from build123d import *

# Parameters (mm, degrees)
CROQUIS1_R                   = 7.65
SALIENTE_EXTRUIR1_DEPTH      = 8.5
CROQUIS2_R                   = 7.65
CROQUIS2_R_2                 = 5
SALIENTE_EXTRUIR2_DEPTH      = 21.5
SALIENTE_EXTRUIR3_REACH      = 132.896
SALIENTE_EXTRUIR3_END_RADIUS = 7.65
SALIENTE_EXTRUIR3_START      = 12
CROQUIS3_R                   = 6.5
CORTAR_EXTRUIR1_REACH        = 129.309
CORTAR_EXTRUIR1_END_RADIUS   = 5
CROQUIS4_R                   = 2.25


with BuildPart() as part:
    # Croquis1 → Saliente-Extruir1 (new, symmetric)
    with BuildSketch(Plane(origin=(0, 0, 0), x_dir=(1, 0, 0), z_dir=(0, 1, 0))):
        with BuildLine():
            ThreePointArc((-18.62950636, 70.733830846), (-21.266037972, 78.379045573), (-29.224003483, 79.818278736))
            ThreePointArc((-29.224003483, 79.818278736), (-42.5, 73.612159322), (-54.51265533, 65.217868785))
            ThreePointArc((-54.51265533, 65.217868785), (-57.245225604, 57.606451909), (-51.942541239, 51.500541191))
            ThreePointArc((-51.942541239, 51.500541191), (-41.569219382, 24), (-70.572047599, 19.233289655))
            ThreePointArc((-70.572047599, 19.233289655), (-78.511263577, 20.772593665), (-83.736658814, 14.600409951))
            ThreePointArc((-83.736658814, 14.600409951), (-85, 0), (-83.736658814, -14.600409951))
            ThreePointArc((-83.736658814, -14.600409951), (-78.511263577, -20.772593665), (-70.572047599, -19.233289655))
            ThreePointArc((-70.572047599, -19.233289655), (-41.569219382, -24), (-51.942541239, -51.500541191))
            ThreePointArc((-51.942541239, -51.500541191), (-57.245225604, -57.606451909), (-54.51265533, -65.217868785))
            ThreePointArc((-54.51265533, -65.217868785), (-42.5, -73.612159322), (-29.224003483, -79.818278736))
            ThreePointArc((-29.224003483, -79.818278736), (-21.266037972, -78.379045573), (-18.62950636, -70.733830846))
            ThreePointArc((-18.62950636, -70.733830846), (0, -48), (18.62950636, -70.733830846))
            ThreePointArc((18.62950636, -70.733830846), (21.266037972, -78.379045573), (29.224003483, -79.818278736))
            ThreePointArc((29.224003483, -79.818278736), (42.5, -73.612159322), (54.51265533, -65.217868785))
            ThreePointArc((54.51265533, -65.217868785), (57.245225604, -57.606451909), (51.942541239, -51.500541191))
            ThreePointArc((51.942541239, -51.500541191), (41.569219382, -24), (70.572047599, -19.233289655))
            ThreePointArc((70.572047599, -19.233289655), (78.511263577, -20.772593665), (83.736658814, -14.600409951))
            ThreePointArc((83.736658814, -14.600409951), (85, 0), (83.736658814, 14.600409951))
            ThreePointArc((83.736658814, 14.600409951), (78.511263577, 20.772593665), (70.572047599, 19.233289655))
            ThreePointArc((70.572047599, 19.233289655), (41.569219382, 24), (51.942541239, 51.500541191))
            ThreePointArc((51.942541239, 51.500541191), (57.245225604, 57.606451909), (54.51265533, 65.217868785))
            ThreePointArc((54.51265533, 65.217868785), (42.5, 73.612159322), (29.224003483, 79.818278736))
            ThreePointArc((29.224003483, 79.818278736), (21.266037972, 78.379045573), (18.62950636, 70.733830846))
            ThreePointArc((18.62950636, 70.733830846), (0, 48), (-18.62950636, 70.733830846))
        make_face()
        with Locations(Location((0, 0, 0), (0, 0, 270))):
            Circle(CROQUIS1_R, mode=Mode.SUBTRACT)
    extrude(amount=SALIENTE_EXTRUIR1_DEPTH, both=True)


with BuildPart() as body_2:
    # Croquis2 → Saliente-Extruir2 (new body)
    with BuildSketch(Plane(origin=(0, 0, 0), x_dir=(1, 0, 0), z_dir=(0, 1, 0))):
        with Locations(Location((0, 0, 0), (0, 0, 270))):
            Circle(CROQUIS2_R)
        with Locations(Location((0, 0, 0), (0, 0, 270))):
            Circle(CROQUIS2_R_2, mode=Mode.SUBTRACT)
    extrude(amount=SALIENTE_EXTRUIR2_DEPTH)

    # Simetría3: body 2 across plane


with BuildPart() as body_2_1:
    add(body_2.part)
    add(body_2.part.mirror(Plane.ZX))

    # Saliente-Extruir3: up to this cylinder (the profile starts outside it)
    saliente_extruir3_end = Plane(origin=(0, 15, 0), z_dir=(0, -1, 0)) * Cylinder(SALIENTE_EXTRUIR3_END_RADIUS, 282.092, mode=Mode.PRIVATE)
    # Croquis3 → Saliente-Extruir3 (add, up to the surface)
    with BuildSketch(Plane.XY.offset(SALIENTE_EXTRUIR3_START), mode=Mode.PRIVATE) as saliente_extruir3_sk1:
        with Locations((0, 15)):
            Circle(CROQUIS3_R)
        Polygon((0, 10.958548116), (3.5, 12.979274058), (3.5, 17.020725942), (0, 19.041451884), (-3.5, 17.020725942), (-3.5, 12.979274058), align=None, mode=Mode.SUBTRACT)
    saliente_extruir3_tool1 = extrude(saliente_extruir3_sk1.sketch, amount=-SALIENTE_EXTRUIR3_REACH, mode=Mode.PRIVATE) - saliente_extruir3_end
    add(saliente_extruir3_tool1.solids().sort_by_distance((-6.316152, 15, 12))[0])

    # Cortar-Extruir1: up to this cylinder (the profile starts outside it)
    cortar_extruir1_end = Plane(origin=(0, 15, 0), z_dir=(0, -1, 0)) * Cylinder(CORTAR_EXTRUIR1_END_RADIUS, 269.618, mode=Mode.PRIVATE)
    # Croquis4 → Cortar-Extruir1 (cut, up to the surface)
    with BuildSketch(Plane.XY.offset(12), mode=Mode.PRIVATE) as cortar_extruir1_sk1:
        with Locations((0, 15)):
            Circle(CROQUIS4_R)
    cortar_extruir1_tool1 = extrude(cortar_extruir1_sk1.sketch, amount=-CORTAR_EXTRUIR1_REACH, mode=Mode.PRIVATE) - cortar_extruir1_end
    add(cortar_extruir1_tool1.solids().sort_by_distance((0, 15, 12))[0], mode=Mode.SUBTRACT)


solid = part.part
Here's how the part is built. I have some questions about the finished solid (model axes, mm). Coordinates: 2 decimals unless noted, no trailing zeros. Order: outer loops, then holes, each group sorted by start corner. A loop starts at its lowest first (then second) coordinate and runs counter-clockwise, first axis right, second up. Notation, with made-up numbers: M -20.75,25.25 L 31.25,25.25 A18 cw 31.25,49.25 Z; hole C 75.5,-13 d11. An arc over 180 degrees is marked long. Answer as CSV lines item,"result".
Item 1: Imagine slicing it at A-A on z = 0. Write out the boundary of the cut face in (x, y).
Results found:
outline,"M -85,-8.5 L -7.65,-8.5 L -7.65,8.5 L -85,8.5 Z; M 7.65,-8.5 L 85,-8.5 L 85,8.5 L 7.65,8.5 Z"
Item 2: We'd pull the mould along X, two halves only. Please class faces 1 (the face through (-42.68, 0.12, 73.51)), 2 (the face through (42.322, 0.119, 73.715)), 3 (the face through (0, 0, -48)): +X half, -X half, draft (parallel to the pull), parting line (faces both ways), or undercut.
Results found:
face 1,"-X half"
face 2,"+X half"
face 3,"undercut"
Item 3: For pin 1 (5 mm diameter, centred on x = 13.5, y = 6, fed in from -Z); pin 2 (23 mm diameter, centred on x = 0, z = 67, fed in from +Y); pin 3 (8 mm diameter, centred on y = 3, z = -18, fed in from -X); pin 4 (1.5 mm diameter, centred on y = -2, z = 45, fed in from +X), each with a flat end and sliding along its axis, tell me the tip position at first contact or that it passes through.
Results found:
pin 1,"z = -56.75"
pin 2,"through"
pin 3,"x = -83.84"
pin 4,"x = 43.5"
Item 4: Imagine slicing it at B-B on x = 0. Write out the boundary of the cut face in (y, z).
Results found:
outline,"M -8.5,-48 L 8.5,-48 L 8.5,-7.65 L -8.5,-7.65 Z; M -8.5,7.65 L 8.5,7.65 L 8.5,48 L -8.5,48 Z"
Item 5: Imagine slicing it at C-C on x = -42. Write out the boundary of the cut face in (y, z), plus the area to 3 significant figures.
Results found:
outline,"M -8.5,-73.9 L 8.5,-73.9 L 8.5,-43.71 L -8.5,-43.71 Z; M -8.5,-23.29 L 8.5,-23.29 L 8.5,23.29 L -8.5,23.29 Z; M -8.5,43.71 L 8.5,43.71 L 8.5,73.9 L -8.5,73.9 Z"
area,"1,820 mm2"
Item 6: Imagine slicing it at D-D on y = 5.75. Write out the boundary of the cut face in (x, z).
Results found:
outline,"M -83.74,-14.6 A8 ccw -70.57,-19.23 A19 cw long -51.94,-51.5 A8 ccw -54.51,-65.22 A85 ccw -29.22,-79.82 A8 ccw -18.63,-70.73 A19 cw long 18.63,-70.73 A8 ccw 29.22,-79.82 A85 ccw 54.51,-65.22 A8 ccw 51.94,-51.5 A19 cw long 70.57,-19.23 A8 ccw 83.74,-14.6 A85 ccw 83.74,14.6 A8 ccw 70.57,19.23 A19 cw long 51.94,51.5 A8 ccw 54.51,65.22 A85 ccw 29.22,79.82 A8 ccw 18.63,70.73 A19 cw long -18.63,70.73 A8 ccw -29.22,79.82 A85 ccw -54.51,65.22 A8 ccw -51.94,51.5 A19 cw long -70.57,19.23 A8 ccw -83.74,14.6 A85 ccw Z; hole C 0,0 d15.3"
Item 7: If I drill on line 1 (Z direction, x = 0.5, y = 1); line 2 (Z direction, x = 50.5, y = 7.5); line 3 (Z direction, x = 43.5, y = 0.5), over which ranges is the centre line in solid material (lowest first)?
Results found:
line 1,"-48.01 to -7.63, 7.63 to 48.01"
line 2,"-68.37 to -50.95, -16.05 to 16.05, 50.95 to 68.37"
line 3,"-73.03 to -45.75, -21.25 to 21.25, 45.75 to 73.03"
